The drawing under review shows one solid part. Ordinate dimensions are in mm from its lowest x, y, z. A direction names the side the tool comes from. Coordinates: 2 decimals unless noted, no trailing zeros. Write each loop counter-clockwise with the first axis right and the second up, starting at its lowest first coordinate (ties: lowest second). Pieces come first, ordered by that corner, then holes.
1) Add section B-B, the plane y = 14.75. State the section outline as (x, z) points.
2) For line 1 (X direction, y = 15.5, z = 1); line 2 (Z direction, x = 28, y = 15); line 3 (Y direction, x = 11, z = 3), list the stretches that pass through material, from the lowest coordinate up.
3) For P1, Ø0.6, axis at x = 3.5, z = 0, coming from the +Y side; P2, Ø6, axis at x = 3, y = 16, coming from the +Z side; P3, Ø2, axis at y = 1, z = 6, coming from the +X side; P4, Ø1, axis at y = 15, z = 5, coming from the +X side, all flat-tipped, find the tip position at first contact; note any pin that passes through.
4) Mouldability with a two-part tool opening along X and no side actions: class the marked faces 3, 4, 5 and 6 as released by +X, released by -X, zero draft, split by the parting line, or undercut.
5) Add section A-A, the plane z = 4.5. State the section outline as (x, y) points, then the cut area to 4 significant figures.
6) Machinability: for the marked faces 1 and 2, which of the approach directions +Z, -Z, +X, -X, +Y, -Y give a long, thin tool a straight path to every point of the face, cutting with its end or side? Answer none if there is none.
7) Add section D-D, the plane y = 11.25. State the section outline as (x, z) points, then the cut area to 3 significant figures.
8) Add section C-C, the plane x = 9. State the section outline as (y, z) points.
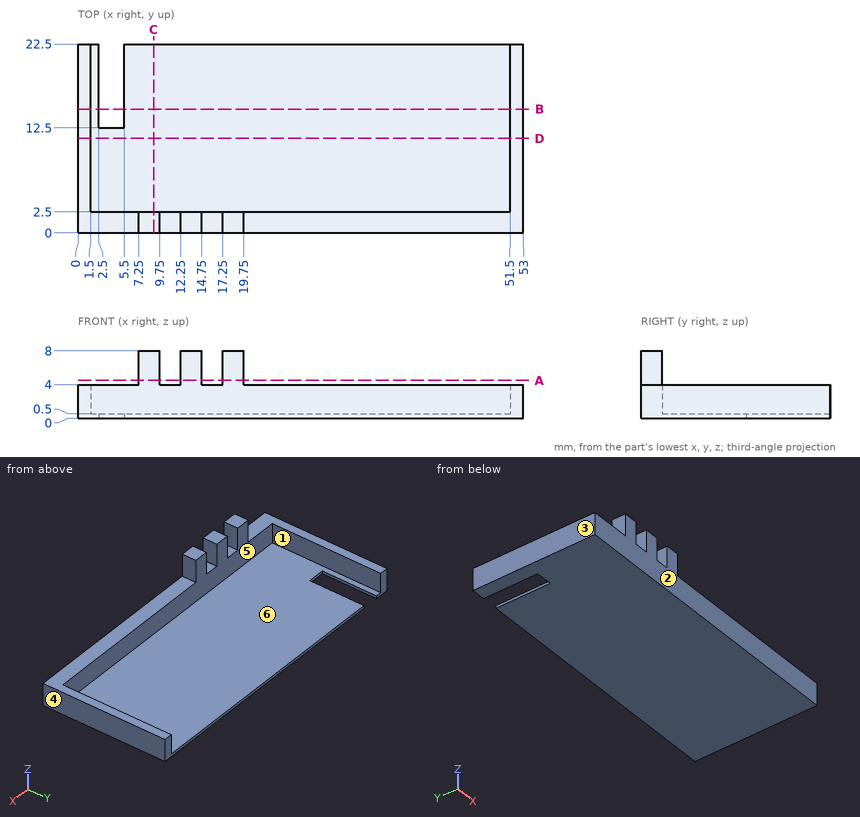
Geometry results:
1. outline: (0, 0) - (2.5, 0) - (2.5, 0.5) - (1.5, 0.5) - (1.5, 4) - (0, 4) - close; (5.5, 0) - (53, 0) - (53, 4) - (51.5, 4) - (51.5, 0.5) - (5.5, 0.5) - close
2. line 1: x = 0 to 1.5, 51.5 to 53
2. line 2: z = 0 to 0.5
2. line 3: y = 0 to 2.5
3. P1: stops at y = 12.5
3. P2: stops at z = 4
3. P3: stops at x = 19.75
3. P4: passes through
4. face 3: released by -X
4. face 4: released by +X
4. face 5: undercut
4. face 6: undercut
5. outline: (7.25, 0) - (9.75, 0) - (9.75, 2.5) - (7.25, 2.5) - close; (12.25, 0) - (14.75, 0) - (14.75, 2.5) - (12.25, 2.5) - close; (17.25, 0) - (19.75, 0) - (19.75, 2.5) - (17.25, 2.5) - close
5. area: 18.75 mm2
6. face 1: +Z, +Y
6. face 2: +Z, -Z, +X, -X, -Y
7. outline: (0, 0) - (53, 0) - (53, 4) - (51.5, 4) - (51.5, 0.5) - (1.5, 0.5) - (1.5, 4) - (0, 4) - close
7. area: 37.0 mm2
8. outline: (0, 0) - (22.5, 0) - (22.5, 0.5) - (2.5, 0.5) - (2.5, 8) - (0, 8) - close
